from build123d import *

# Parameters (mm, degrees)
SKETCH_1_R          = 11
SKETCH_1_R_2        = 2.5
EXTRUDE_1_DEPTH     = 3
SKETCH_2_R          = 1.5
CUT_EXTRUDE_1_DEPTH = 401.392640069
SKETCH_3_R          = 1.5
CUT_EXTRUDE_2_DEPTH = 10
SKETCH_4_R          = 1.494410779
SKETCH_4_R_2        = 1.5
CUT_EXTRUDE_3_DEPTH = 615.946278901
SKETCH_6_R          = 5
CUT_EXTRUDE_5_DEPTH = 401.392640069


with BuildPart() as part:
    # 草图1 → 凸台-拉伸1 (new body)
    with BuildSketch(Plane(origin=(0, 0, 0), x_dir=(1, 0, 0), z_dir=(0, 1, 0))):
        Polygon((68.894458013, 60.758817204), (86.717926663, 82), (374.070989363, 82), (391.894458013, 60.758817204), (391.894458013, 0), (68.894458013, 0), align=None)
        with Locations(Location((135.394458013, 27, 0), (0, 0, 270))):
            Circle(SKETCH_1_R, mode=Mode.SUBTRACT)
        with Locations(Location((311.394458013, 27, 0), (0, 0, 90))):
            Circle(SKETCH_1_R_2, mode=Mode.SUBTRACT)
        with Locations(Location((339.394458013, 27, 0), (0, 0, 90))):
            Circle(SKETCH_1_R_2, mode=Mode.SUBTRACT)
        with Locations(Location((325.394458013, 27, 0), (0, 0, 90))):
            Circle(SKETCH_1_R, mode=Mode.SUBTRACT)
        with Locations(Location((121.394458013, 27, 0), (0, 0, 270))):
            Circle(SKETCH_1_R_2, mode=Mode.SUBTRACT)
        with Locations(Location((149.394458013, 27, 0), (0, 0, 270))):
            Circle(SKETCH_1_R_2, mode=Mode.SUBTRACT)
    extrude(amount=EXTRUDE_1_DEPTH)

    # 草图2 → 切除-拉伸1 (cut, through all)
    with BuildSketch(Plane(origin=(0, 3, 0), x_dir=(1, 0, 0), z_dir=(0, 1, 0))):
        with Locations(Location((236.394458013, 10.5, 0), (0, 0, 270))):
            Circle(SKETCH_2_R)
        with Locations(Location((353.894458013, 10.5, 0), (0, 0, 270))):
            Circle(SKETCH_2_R)
        with Locations(Location((365.894458013, 10.5, 0), (0, 0, 270))):
            Circle(SKETCH_2_R)
        with Locations(Location((381.394458013, 6, 0), (0, 0, 270))):
            Circle(SKETCH_2_R)
        with Locations(Location((381.394458013, 18, 0), (0, 0, 270))):
            Circle(SKETCH_2_R)
        with Locations(Location((79.394458013, 18, 0), (0, 0, 90))):
            Circle(SKETCH_2_R)
        with Locations(Location((79.394458013, 6, 0), (0, 0, 90))):
            Circle(SKETCH_2_R)
        with Locations(Location((94.894458013, 10.5, 0), (0, 0, 90))):
            Circle(SKETCH_2_R)
        with Locations(Location((106.894458013, 10.5, 0), (0, 0, 90))):
            Circle(SKETCH_2_R)
        with Locations(Location((224.394458013, 10.5, 0), (0, 0, 90))):
            Circle(SKETCH_2_R)
    extrude(amount=-CUT_EXTRUDE_1_DEPTH, mode=Mode.SUBTRACT)

    # 草图3 → 切除-拉伸2 (cut)
    with BuildSketch(Plane(origin=(0, 3, 0), x_dir=(1, 0, 0), z_dir=(0, 1, 0))):
        with Locations(Location((248.894458013, 32, 0), (0, 0, 270))):
            Circle(SKETCH_3_R)
        with Locations(Location((211.894458013, 32, 0), (0, 0, 270))):
            Circle(SKETCH_3_R)
    extrude(amount=-CUT_EXTRUDE_2_DEPTH, mode=Mode.SUBTRACT)

    # 草图4 → 切除-拉伸3 (cut, through all)
    with BuildSketch(Plane(origin=(-213.132295014, -49, -96.940982333), x_dir=(1, 0, 0), z_dir=(0, -1, 0))):
        with Locations((449.526753027, 18.940982333)):
            Circle(SKETCH_4_R)
        with Locations((437.526753027, 18.940982333)):
            Circle(SKETCH_4_R_2)
        with Locations((562.026753027, 18.940982333)):
            Circle(SKETCH_4_R_2)
        with Locations((574.026753027, 18.940982333)):
            Circle(SKETCH_4_R_2)
        with Locations((325.026753027, 18.940982333)):
            Circle(SKETCH_4_R_2)
        with Locations((313.026753027, 18.940982333)):
            Circle(SKETCH_4_R_2)
    extrude(amount=-CUT_EXTRUDE_3_DEPTH, mode=Mode.SUBTRACT)

    # 草图6 → 切除-拉伸5 (cut, through all)
    with BuildSketch(Plane(origin=(0, 3, 0), x_dir=(1, 0, 0), z_dir=(0, 1, 0))):
        with Locations(Location((230.394458013, 52, 0), (0, 0, 270))):
            Circle(SKETCH_6_R)
    extrude(amount=-CUT_EXTRUDE_5_DEPTH, mode=Mode.SUBTRACT)


solid = part.part
Can you work these out from the model? Positions are in its coordinate system, mm. Give positions to 0.01 mm unless a question says otherwise; leave off trailing zeros. Use one line per item in the form item = value. Start each with the question number.
Item 1: We'd pull the mould along Z, two halves only. Please class faces 1 (the flat face through (233, 0, -42)), 2 (the cylindrical face through (235.352, 1.521, -52.651)), 3 (the flat face through (382.858, 1.479, -71.528)): +Z half, -Z half, draft (parallel to the pull), parting line (faces both ways), or undercut.
Item 2: If we section it at A-A (y = 2): State how many separate pieces and enclosed holes the cut face has, then the cut area to 3 significant figures.
Item 3: If I drill on line 1 along X through (y, z) = (2.45, -6); line 2 along Z through (x, y) = (224.5, 1.4); line 3 along Z through (x, y) = (225, 2.4), over which ranges is the centre line in solid material (lowest first)?
Item 4: Will this pin go through, and if not, where does the flat tip stop? pin 1 Ø3 at (x, z) = (149.39, -27) entering from -Y.
Outcome:
q1.face_1 = draft
q1.face_2 = undercut
q1.face_3 = -Z half
q2.separate_pieces = 1
q2.enclosed_holes = 25
q2.area = 25,100 mm2
q3.line_1 = 68.89 to 77.89, 80.89 to 379.89, 382.89 to 391.89
q3.line_2 = -82 to -79.5, -76.5 to -12, -9 to 0
q3.line_3 = -82 to -79.37, -76.63 to -11.87, -9.13 to 0
q4.pin_1 = through
